Read the model definition and answer for the solid it produces. Units are mm, in the model's axes. A direction names the side the tool comes from. Give positions to 0.01 mm unless a question says otherwise; leave off trailing zeros. Write each loop counter-clockwise with the first axis right and the second up, starting at its lowest first coordinate (ties: lowest second). Pieces come first, ordered by that corner, then holes. Notation, with made-up numbers: (69.5, -6.5) - (75.5, -6.5) arc R20 cw to (75.5, 12.5) - close; hole circle Ø4 at (-6.5, 56.5). An arc over 180 degrees is marked (long way). Use CSV: the item, a comma, the result in double quotes. Start each with the question number.
from build123d import *


with BuildPart() as part:
    # Sketch1 → Revolve1 (revolve)
    with BuildSketch(Plane(origin=(0, 0, 0), x_dir=(0, 0, -1), z_dir=(1, 0, 0))):
        with BuildLine():
            Line((-12.5, 1.6), (-12.5, 5.699104428))
            ThreePointArc((-12.5, 5.699104428), (-12.457637435, 5.823900521), (-12.348057904, 5.897119222))
            Line((-12.348057904, 5.897119222), (-4.5, 8))
            Line((-4.5, 8), (0.295, 8))
            ThreePointArc((0.295, 8), (0.43995689, 7.93995689), (0.5, 7.795))
            Line((0.5, 7.795), (0.5, 4.615))
            ThreePointArc((0.5, 4.615), (0.35504311, 4.55495689), (0.295, 4.41))
            Line((0.295, 4.41), (0.295, 4))
            ThreePointArc((0.295, 4), (0.35504311, 3.85504311), (0.5, 3.795))
            Line((0.5, 3.795), (1.525, 3.795))
            Line((1.525, 3.795), (1.73, 4))
            Line((1.73, 4), (10.45, 4))
            Line((10.45, 4), (12.348057904, 3.491416917))
            ThreePointArc((12.348057904, 3.491416917), (12.457637435, 3.418198216), (12.5, 3.293402123))
            Line((12.5, 3.293402123), (12.5, 0))
            Line((12.5, 0), (-11.8372583, 0))
            Line((-11.8372583, 0), (-12.5, 1.6))
        make_face()
    revolve(axis=Axis((0, 0, -12.5), (0, 0, 1)))


solid = part.part
(1) Consider probe 1 along X at (y, z) = (1.5, -1); probe 2 along Z at (x, y) = (-5.25, 1); probe 3 along X at (y, z) = (-2, 11). Determine where each line is inside the solid, lowest interval first.
(2) The part is cut by section B-B on z = -2. Write down the section's boundary in (x, y).
(3) The part is cut by section A-A on z = 2.5. Write down the section's boundary in (x, y).
(4) Which of the six approach directions +Z, -Z, +X, -X, +Y, -Y give full straight-line access (tool end or side, diameter ignored) to faces 5 (the face through (6.34, -1.41, 10.11)), 6 (the face through (3.4, 3.4, -0.5))?
(5) Given P1, Ø6, axis at y = -4, z = -2, coming from the +X side; P2, Ø2, axis at x = 3, z = 2.5, coming from the +Y side; P3, Ø1, axis at y = 0.5, z = -9, coming from the +X side, each flat-ended and moving along its own axis, determine where each tip first touches the part or whether it passes through.
(6) For a pull along Z with two mould halves and no side action, classify faces 1 (the face through (0, 0, -12.5)), 2 (the face through (3.905, -0.867, -6.151)), 3 (the face through (1.454, 3.506, -1.02)), 4 (the face through (-0.03, 0.1, 11.88)) as pulls with the +Z half, pulls with the -Z half, needs draft (parallel to the pull), parting line crosses it, or undercut.
Reported:
1,probe 1,"-3.49 to 3.49"
1,probe 2,"-0.5 to 12.5"
1,probe 3,"-5.93 to 5.93"
2,outline,"circle Ø8 at (0, 0)"
3,outline,"circle Ø16 at (0, 0)"
4,face 5,"+Z"
4,face 6,"-Z"
5,P1,"x = 7.85"
5,P2,"y = 7.75"
5,P3,"x = 4"
6,face 1,"pulls with the -Z half"
6,face 2,"needs draft"
6,face 3,"undercut"
6,face 4,"pulls with the +Z half"
